For this review, take the finished solid that the model builds, in its own axes (mm). Face numbers are marked on the shaded views. A direction names the side the tool comes from. Give positions to 0.01 mm unless a question says otherwise; leave off trailing zeros. Order: outer loops, then holes, each group sorted by start corner. A loop starts at its lowest first (then second) coordinate and runs counter-clockwise, first axis right, second up.
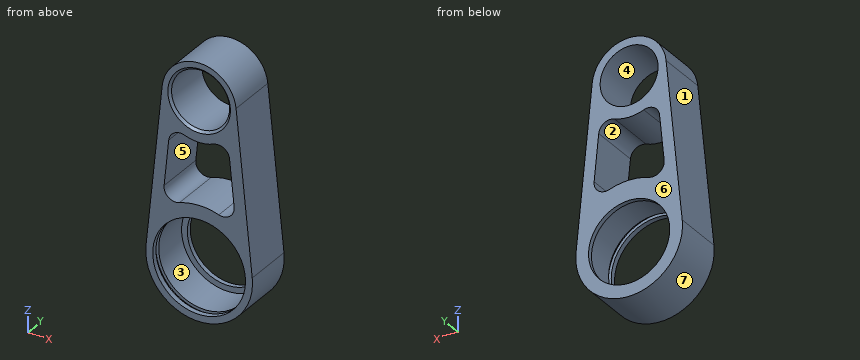
from build123d import *

# Parameters (mm, degrees)
F0_R           = 12.5
F1_DEPTH       = 22
F2_SIZE        = 1
F4_D           = 35
F4_CBORE_D     = 40
F4_CBORE_DEPTH = 20
F5_W           = 1.85
F5_H           = 21.25


with BuildPart() as f1:
    # F0 (on Front) → F1 (new body)
    with BuildSketch(Plane.XZ):
        with BuildLine():
            Line((-15.919799, 71.6), (-22.884711, 2.3))
            ThreePointArc((-22.884711, 2.3), (0, -23), (22.884711, 2.3))
            Line((22.884711, 2.3), (15.919799, 71.6))
            ThreePointArc((15.919799, 71.6), (0, 86), (-15.919799, 71.6))
        make_face()
        with BuildLine():
            ThreePointArc((-13.113387, 49.52345), (-10.753012, 53.285382), (-6.329905, 53.684906))
            ThreePointArc((-6.329905, 53.684906), (0, 52.5), (6.329905, 53.684906))
            ThreePointArc((6.329905, 53.684906), (10.753012, 53.285382), (13.113387, 49.52345))
            Line((13.113387, 49.52345), (15.095524, 29.801429))
            ThreePointArc((15.095524, 29.801429), (13.222374, 25.379832), (8.488234, 24.575392))
            ThreePointArc((8.488234, 24.575392), (0, 26), (-8.488234, 24.575392))
            ThreePointArc((-8.488234, 24.575392), (-13.222374, 25.379832), (-15.095524, 29.801429))
            Line((-15.095524, 29.801429), (-13.113387, 49.52345))
        make_face(mode=Mode.SUBTRACT)
        with Locations((0, 70)):
            Circle(F0_R, mode=Mode.SUBTRACT)
    extrude(amount=F1_DEPTH)

    # F2
    f2_edges = [f1.edges().sort_by_distance(p)[0] for p in [
        (-12.5, -22, 70),
    ]]
    chamfer(f2_edges, length=F2_SIZE)

    # F4 (through all)
    with Locations(Plane.XZ.offset(22)):
        with Locations((0, 0)):
            CounterBoreHole(F4_D / 2, F4_CBORE_D / 2, F4_CBORE_DEPTH)

    # F5 (on Right) → F6 (revolve, cut)
    with BuildSketch(Plane.YZ):
        with Locations((-18.825, 10.625)):
            Rectangle(F5_W, F5_H)
    revolve(axis=Axis((0, -18.825, 0), (0, -1, 0)), mode=Mode.SUBTRACT)


solid = f1.part
1) To check wall thickness, follow line 1 (Z direction, x = -0.5, y = -18.25); line 2 (Z direction, x = 0, y = -0.95); line 3 (X direction, y = -19, z = 0). State the ranges of each line that lie inside material, in increasing order.
Answer sheet:
line 1: z = -22.99 to -21.24, 21.24 to 26, 52.51 to 57.51, 82.49 to 85.99
line 2: z = -23 to -17.5, 17.5 to 26, 52.5 to 57.5, 82.5 to 86
line 3: x = -23 to -21.25, 21.25 to 23
2) Draft analysis for pull direction X (two halves, no side actions). For the marked faces 4, 5, 6 and 7, state which applies: +X half, -X half, draft (parallel to the pull), parting line (faces both ways), or undercut.
Answer sheet:
face 4: undercut
face 5: undercut
face 6: draft
face 7: parting line
3) We need section C-C on y = -14.25. Give the boundary of the cut face in (x, z), then the cut area to 3 significant figures.
Answer sheet:
outline: (-22.88, 2.3) arc R23 ccw (long way) to (22.88, 2.3) - (15.92, 71.6) arc R16 ccw to (-15.92, 71.6) - close; hole circle Ø40 at (0, 0); hole (-15.1, 29.8) arc R5 ccw to (-8.49, 24.58) arc R26 cw to (8.49, 24.58) arc R5 ccw to (15.1, 29.8) - (13.11, 49.52) arc R5 ccw to (6.33, 53.68) arc R17.5 cw to (-6.33, 53.68) arc R5 ccw to (-13.11, 49.52) - close; hole circle Ø25 at (0, 70)
area: 1,450 mm2
4) We need section A-A on z = 0. Give the boundary of the cut face in (x, y), then the cut area to 3 significant figures.
Answer sheet:
outline: (-23, -22) - (-20, -22) - (-20, -19.75) - (-21.25, -19.75) - (-21.25, -17.9) - (-20, -17.9) - (-20, -2) - (-17.5, -2) - (-17.5, 0) - (-23, 0) - close; (17.5, -2) - (20, -2) - (20, -17.9) - (21.25, -17.9) - (21.25, -19.75) - (20, -19.75) - (20, -22) - (23, -22) - (23, 0) - (17.5, 0) - close
area: 137 mm2
5) We need section D-D on x = 18.5. Give the boundary of the cut face in (y, z).
Answer sheet:
outline: (-22, -13.67) - (0, -13.67) - (0, 45.93) - (-22, 45.93) - (-22, 7.6) - (-19.75, 7.6) - (-19.75, 10.46) - (-17.9, 10.46) - (-17.9, 7.6) - (-2, 7.6) - (-2, -7.6) - (-17.9, -7.6) - (-17.9, -10.46) - (-19.75, -10.46) - (-19.75, -7.6) - (-22, -7.6) - close
6) Clearance check with flat-ended pins moving along their axes: pin 1 (8 mm diameter, centred on y = -19.5, z = 11.5, fed in from -X); pin 2 (21 mm diameter, centred on x = 0, z = 0, fed in from +Y); pin 3 (1.5 mm diameter, centred on x = 13, y = -2.5, fed in from -Z); pin 4 (10 mm diameter, centred on x = -6.5, y = -19.5, fed in from -Z). State where each tip first meets the part, or that it passes through.
Answer sheet:
pin 1: stops at x = -22.36
pin 2: passes through
pin 3: stops at z = -19.47
pin 4: stops at z = -22.95
7) We need section B-B on x = 0. Count the separate pieces of the cut face and the enclosed holes in it, then the cut area to 3 significant figures.
Answer sheet:
separate pieces: 4
enclosed holes: 0
area: 389 mm2
8) Tool access review of the marked faces 1, 2 and 3: name each direction out of +Z, -Z, +X, -X, +Y, -Y from which nothing blocks a thin tool from reaching the whole face with its end or side.
Answer sheet:
face 1: +Z, -X, +Y, -Y
face 2: +Y, -Y
face 3: -Y
